from build123d import *

# Parameters (mm, degrees)
F0_W     = 50
F0_H     = 50
F1_DEPTH = 2
F2_R     = 2
F3_DEPTH = 2
F4_W     = 14
F4_H     = 20
F5_DEPTH = 1
F6_W     = 2.9
F6_H     = 10
F7_DEPTH = 14.5
F8_R     = 4.99999


# Not quite as in the source:
# - a fillet or chamfer is up to 0.001 mm smaller than in the source, because OpenCascade refuses the exact size


with BuildPart() as f1:
    # F0 (on Top) → F1 (new body)
    with BuildSketch(Plane.XY):
        Rectangle(F0_W, F0_H)
    extrude(amount=F1_DEPTH)

    # F2 (on face) → F3 (cut)
    with BuildSketch(Plane.XY.offset(2)):
        with Locations((-20.25, 20.25)):
            Circle(F2_R)
        with Locations((20.25, 20.25)):
            Circle(F2_R)
        with Locations((20.25, -20.25)):
            Circle(F2_R)
        with Locations((-20.25, -20.25)):
            Circle(F2_R)
    extrude(amount=-F3_DEPTH, mode=Mode.SUBTRACT)

    # F4 (on face) → F5 (join)
    with BuildSketch(Plane.XY.offset(2)):
        Rectangle(F4_W, F4_H)
    extrude(amount=F5_DEPTH)

    # F6 (on face) → F7 (join)
    with BuildSketch(Plane.XY.offset(3)):
        with Locations((3.05, 0)):
            Rectangle(F6_W, F6_H)
        with Locations((-3.05, 0)):
            Rectangle(F6_W, F6_H)
    extrude(amount=F7_DEPTH)

    # F8 (radius 5 in the source; OpenCascade refuses exactly that, so slightly less here)
    f8_edges = [f1.edges().sort_by_distance(p)[0] for p in [
        (-3.05, 5, 17.5),
        (3.05, 5, 17.5),
        (3.05, -5, 17.5),
        (-3.05, -5, 17.5),
    ]]
    fillet(f8_edges, radius=F8_R)


solid = f1.part
CAD build for the part. Positions are in the model's coordinates, mm. A direction names the side the tool comes from. Round coordinates to 2 decimals unless told otherwise and drop trailing zeros. Write each loop counter-clockwise with the first axis right and the second up, starting at its lowest first coordinate (ties: lowest second). Pieces come first, ordered by that corner, then holes. Notation, with made-up numbers: M 49.5,35 L 78.5,35 A12 cw 78.5,48 Z; hole C -5.5,-22.75 d5. An arc over 180 degrees is marked long. Put each result on its own line as item: value. Start each with the question number.
1) Saw through at A-A, the plane y = -20.25. Write the cut outline in (x, z), and give its area (3 significant figures).
2) Drill centre lines: probe 1 along Y at (x, z) = (-20.25, 1.4); probe 2 along X at (y, z) = (-3.5, 10.5); probe 3 along Z at (x, y) = (-5, -4). Where is each one in solid material? Low to high. Write a range as [from, to].
3) Saw through at C-C, the plane z = 7. Write the cut outline in (x, y), and give its area (3 significant figures).
4) Saw through at D-D, the plane y = 15. Write the cut outline in (x, z), and give its area (3 significant figures).
5) Pull direction Y, two halves, no side cores. Call faces 4 (the flat face through (3, 5, 8)), 5 (the cylindrical face through (-20.51, -18.267, 1.014)), 6 (the cylindrical face through (-3.03, -3.57, 16)), 7 (the cylindrical face through (19.99, 22.233, 1.014)): pulls with the +Y half, pulls with the -Y half, needs draft (parallel to the pull), parting line crosses it, or undercut.
6) Pin check, flat tips, straight feed: pin 1 Ø2 at (x, y) = (-9.5, 14.5) entering from +Z; pin 2 Ø3 at (x, y) = (-20.25, -20.25) entering from +Z; pin 3 Ø3 at (y, z) = (2.5, 12) entering from +X; pin 4 Ø1 at (x, y) = (-4, 2) entering from +Z. Stop position of each tip, or through.
7) 3-axis set-ups, long thin cutter, end or side, ignore diameter. For faces 1 (the flat face through (3, -5, 8)), 2 (the flat face through (-3, 5, 8)), 3 (the flat face through (-4.5, 0, 10)): which of +Z, -Z, +X, -X, +Y, -Y reach the whole face in a straight line?
Resolved:
1. outline: M -25,0 L -22.25,0 L -22.25,2 L -25,2 Z; M -18.25,0 L 18.25,0 L 18.25,2 L -18.25,2 Z; M 22.25,0 L 25,0 L 25,2 L 22.25,2 Z
1. area: 84.0 mm²
2. probe 1: [-25, -22.25], [-18.25, 18.25], [22.25, 25]
2. probe 2: [-4.5, -1.6], [1.6, 4.5]
2. probe 3: [0, 3]
3. outline: M -4.5,-5 L -1.6,-5 L -1.6,5 L -4.5,5 Z; M 1.6,-5 L 4.5,-5 L 4.5,5 L 1.6,5 Z
3. area: 58.0 mm²
4. outline: M -25,0 L 25,0 L 25,2 L -25,2 Z
4. area: 100 mm²
5. face 4: pulls with the +Y half
5. face 5: undercut
5. face 6: pulls with the -Y half
5. face 7: undercut
6. pin 1: z = 2
6. pin 2: through
6. pin 3: x = 4.5
6. pin 4: z = 17.27
7. face 1: +Z, +X, -X, -Y
7. face 2: +Z, +X, -X, +Y
7. face 3: +Z, -X, +Y, -Y
